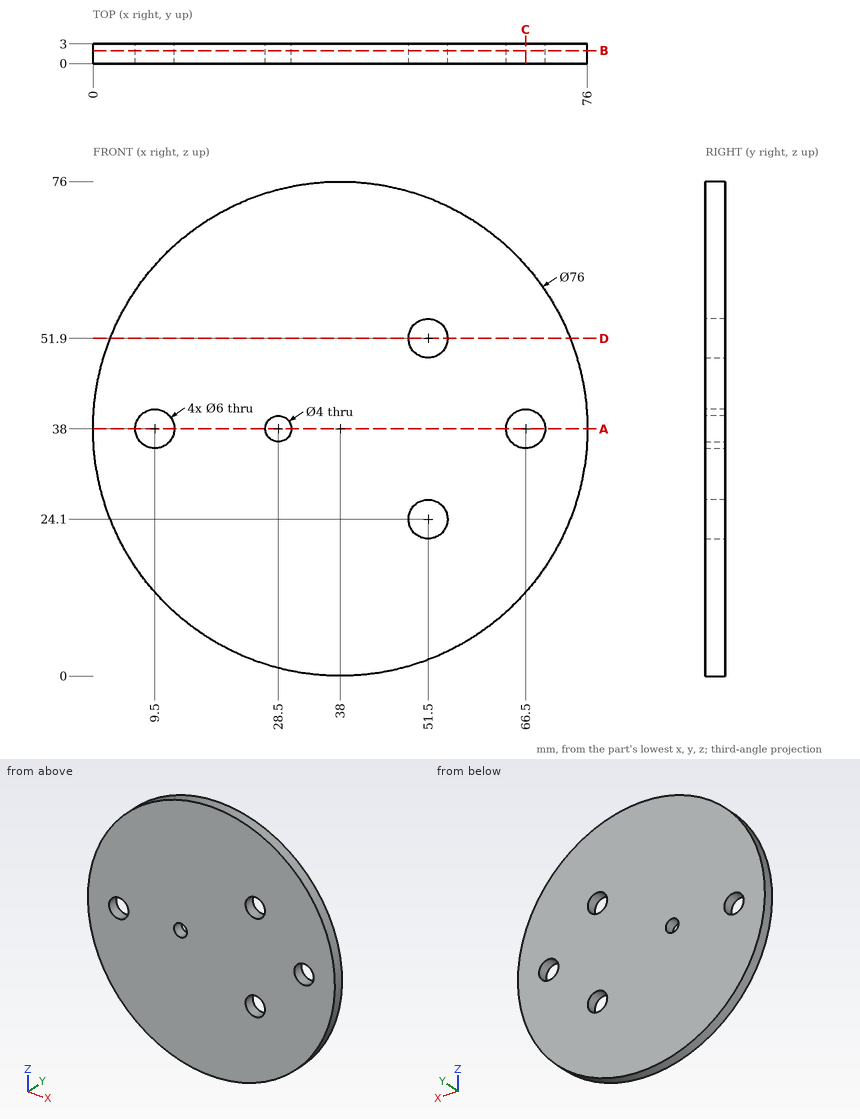
For this review, use the dimensioned drawing (mm, ordinates from the lowest corner) and the shaded views. Coordinates: 2 decimals unless noted, no trailing zeros. Loops run counter-clockwise (first coordinate to the right, second up) from the corner with the lowest first, then second, coordinate; pieces in that order, holes last.
1. Add section C-C, the plane x = 66.5. Give the boundary of the cut face in (y, z), then the cut area to 3 significant figures.
2. Add section B-B, the plane y = 2. Give the boundary of the cut face in (x, z).
3. Add section A-A, the plane z = 38. Give the boundary of the cut face in (x, y).
4. For line 1 (X direction, y = 1.6, z = 38); line 2 (X direction, y = 0.7, z = 51); line 3 (X direction, y = 1.1, z = 51.9), list the stretches that pass through material, from the lowest coordinate up.
5. Add section D-D, the plane z = 51.9. Give the boundary of the cut face in (x, y), then the cut area to 3 significant figures.
6. Insertion check: P1, Ø7, axis at x = 51.5, z = 51.9, coming from the +Y side. The pin has a flat end and moves straight along its axis. Give the tip position at first contact, or say it passes through.
Result:
1. outline: (0, 12.87) - (3, 12.87) - (3, 35) - (0, 35) - close; (0, 41) - (3, 41) - (3, 63.13) - (0, 63.13) - close
1. area: 133 mm2
2. outline: circle Ø76 at (38, 38); hole circle Ø6 at (9.5, 38); hole circle Ø4 at (28.5, 38); hole circle Ø6 at (51.5, 24.1); hole circle Ø6 at (51.5, 51.9); hole circle Ø6 at (66.5, 38)
3. outline: (0, 0) - (6.5, 0) - (6.5, 3) - (0, 3) - close; (12.5, 0) - (26.5, 0) - (26.5, 3) - (12.5, 3) - close; (30.5, 0) - (63.5, 0) - (63.5, 3) - (30.5, 3) - close; (69.5, 0) - (76, 0) - (76, 3) - (69.5, 3) - close
4. line 1: x = 0 to 6.5, 12.5 to 26.5, 30.5 to 63.5, 69.5 to 76
4. line 2: x = 2.29 to 48.64, 54.36 to 73.71
4. line 3: x = 2.63 to 48.5, 54.5 to 73.37
5. outline: (2.63, 0) - (48.5, 0) - (48.5, 3) - (2.63, 3) - close; (54.5, 0) - (73.37, 0) - (73.37, 3) - (54.5, 3) - close
5. area: 194 mm2
6. P1: stops at y = 3
